Model file for the job. Use its own axes, mm. A direction names the side the tool comes from. Round coordinates to 2 decimals unless told otherwise and drop trailing zeros. Order: outer loops, then holes, each group sorted by start corner. A loop starts at its lowest first (then second) coordinate and runs counter-clockwise, first axis right, second up. Notation, with made-up numbers: (38, 14) - (48, 14) arc R23 ccw to (48, 23) - close; hole circle Ø5 at (-33.75, -18.5). An arc over 180 degrees is marked (long way). Use one line per item in the form item = value.
from build123d import *

# Parameters (mm, degrees)
SKETCH1_W                     = 55
SKETCH1_H                     = 11.85
BOSS_EXTRUDE1_DEPTH           = 4.25
CHAMFER1_SIZE                 = 0.5
BOSS_EXTRUDE2_DEPTH           = 27
BOSS_EXTRUDE2_DEPTH_BACK      = 27
SKETCH7_W                     = 5.5
SKETCH7_H                     = 2.15
CBORE_FOR_M3_SHCS1_AT_2_COUNT = 2
CBORE_FOR_M3_SHCS1_AT_2_PITCH = 45
BOSS_EXTRUDE3_DEPTH           = 9
CUT_EXTRUDE1_DEPTH            = 2
CUT_EXTRUDE1_DEPTH_BACK       = 2
SKETCH10_W                    = 3.3
SKETCH10_H                    = 2.5


with BuildPart() as part:
    # Sketch1 → Boss-Extrude1 (new body)
    with BuildSketch(Plane(origin=(0, 0, 0), x_dir=(1, 0, 0), z_dir=(0, 1, 0))):
        Rectangle(SKETCH1_W, SKETCH1_H)
    extrude(amount=BOSS_EXTRUDE1_DEPTH)

    # Chamfer1
    chamfer1_edges = [part.edges().sort_by_distance(p)[0] for p in [
        (-27.5, 4.25, 0),
        (0, 4.25, 5.925),
        (0, 0, 5.925),
        (-27.5, 0, 0),
        (0, 0, -5.925),
        (-27.5, 2.125, 5.925),
        (-27.5, 2.125, -5.925),
        (0, 4.25, -5.925),
    ]]
    chamfer(chamfer1_edges, length=CHAMFER1_SIZE)

    # Sketch7 → Boss-Extrude2 (add, two sides: drawn at the far end of the back side and taken through both)
    with BuildSketch(Plane(origin=(0, 0, 0), x_dir=(0, 0, -1), z_dir=(1, 0, 0)).offset(-BOSS_EXTRUDE2_DEPTH_BACK)):
        with Locations((0, 5.325)):
            Rectangle(SKETCH7_W, SKETCH7_H)
    extrude(amount=BOSS_EXTRUDE2_DEPTH + BOSS_EXTRUDE2_DEPTH_BACK)

    # Sketch6 → CBORE for M3 SHCS1 (revolve, cut)
    with BuildSketch(Plane(origin=(22.5, 0, 0), x_dir=(0, 0, -1), z_dir=(1, 0, 0))):
        Polygon((0, 0), (0, 6.4), (1.8, 6.4), (1.8, 2.2), (3.25, 2.2), (3.25, 0.025), (3.275, 0), align=None)
    cbore_for_m3_shcs1 = revolve(axis=Axis((22.5, -6.35, 0), (0, 1, 0)), mode=Mode.SUBTRACT)

    # CBORE for M3 SHCS1 at 2: CBORE for M3 SHCS1 ×2
    with Locations(*[(-i * CBORE_FOR_M3_SHCS1_AT_2_PITCH, 0, 0) for i in range(1, CBORE_FOR_M3_SHCS1_AT_2_COUNT)]):
        add(cbore_for_m3_shcs1, mode=Mode.SUBTRACT)

    # Sketch8 → Boss-Extrude3 (add)
    with BuildSketch(Plane(origin=(27.5, 0, 0), x_dir=(0, 0, -1), z_dir=(1, 0, 0))):
        Polygon((5.425, 4.25), (-5.425, 4.25), (-5.925, 3.75), (-5.925, 0.5), (-5.425, 0), (5.425, 0), (5.925, 0.5), (5.925, 3.75), align=None)
    extrude(amount=BOSS_EXTRUDE3_DEPTH)

    # Sketch10 → Cut-Extrude1 (cut, two sides: drawn at the far end of the back side and taken through both)
    with BuildSketch(Plane.XY.offset(-CUT_EXTRUDE1_DEPTH_BACK)):
        with Locations((32.8, 1.25)):
            Rectangle(SKETCH10_W, SKETCH10_H)
    extrude(amount=CUT_EXTRUDE1_DEPTH + CUT_EXTRUDE1_DEPTH_BACK, mode=Mode.SUBTRACT)


solid = part.part
(1) Pin check, flat tips, straight feed: pin 1 (0.6 mm diameter, centred on y = 5.5, z = 0, fed in from -X); pin 2 (6 mm diameter, centred on x = -22.5, z = 0, fed in from -Y); pin 3 (6 mm diameter, centred on x = -7, z = -3, fed in from +Y); pin 4 (3 mm diameter, centred on x = 22.5, z = 0, fed in from +Y). Stop position of each tip, or through.
Report:
pin_1 = -27
pin_2 = 2.2
pin_3 = 6.4
pin_4 = through
(2) Probe probe 1 along X at (y, z) = (0.5, 0); probe 2 along X at (y, z) = (4.6, 0); probe 3 along Z at (x, y) = (22.5, 3.2) (3 decimals). List the from-to ranges inside material, lowest first. Write a range as [from, to].
Report:
probe_1 = [-27.5, -25.75], [-19.25, 19.25], [25.75, 31.15], [34.45, 36.5]
probe_2 = [-27, -24.3], [-20.7, 20.7], [24.3, 27]
probe_3 = [-5.925, -1.8], [1.8, 5.925]
(3) Slice it at B-B on z = 0. Count the separate pieces of the cut face and the enclosed holes in it, then the cut area to 3 significant figures.
Report:
separate_pieces = 3
enclosed_holes = 0
area = 321 mm2
(4) Slice it at C-C on x = 4. Give the cut face in (y, z) (3 decimals), then the cut area to 3 significant figures.
Report:
outline = (0, -5.425) - (0.5, -5.925) - (3.75, -5.925) - (4.25, -5.425) - (4.25, -2.75) - (6.4, -2.75) - (6.4, 2.75) - (4.25, 2.75) - (4.25, 5.425) - (3.75, 5.925) - (0.5, 5.925) - (0, 5.425) - close
area = 61.7 mm2
(5) Pull direction X, two halves, no side cores. Call faces 1 (the face through (0, 6.4, 0)), 2 (the face through (33, 1, 2)), 3 (the face through (36.5, 2, 0)): released by +X, released by -X, zero draft, split by the parting line, or undercut.
Report:
face_1 = zero draft
face_2 = undercut
face_3 = released by +X
(6) Slice it at A-A on x = -22.5. Give the cut face in (y, z) (3 decimals), then the cut area to 3 significant figures.
Report:
outline = (0, -5.425) - (0.5, -5.925) - (3.75, -5.925) - (4.25, -5.425) - (4.25, -2.75) - (6.4, -2.75) - (6.4, -1.8) - (2.2, -1.8) - (2.2, -3.25) - (0.025, -3.25) - (0, -3.275) - close; (0, 3.275) - (0.025, 3.25) - (2.2, 3.25) - (2.2, 1.8) - (6.4, 1.8) - (6.4, 2.75) - (4.25, 2.75) - (4.25, 5.425) - (3.75, 5.925) - (0.5, 5.925) - (0, 5.425) - close
area = 32.3 mm2
(7) Tool access for faces 4 (the face through (0, 5, 2.75)), 5 (the face through (0, 5, -2.75)), 6 (the face through (27, 5, 0)), 7 (the face through (-21.1, 2.2, 1.4)): list every direction of +Z, -Z, +X, -X, +Y, -Y with a clear straight run to the whole face (end or side of a thin tool).
Report:
face_4 = +Z, +X, -X, +Y
face_5 = -Z, +X, -X, +Y
face_6 = +Z, -Z, +X, +Y
face_7 = -Y
